from build123d import *

# Parameters (mm, degrees)
F1_DEPTH = 3.2
F2_R     = 14.060754
F3_DEPTH = 2


with BuildPart() as f1:
    # F0 (on Top) → F1 (new body)
    with BuildSketch(Plane.XY):
        with BuildLine():
            ThreePointArc((-5.086545, -8.556186), (-9.186545, 0.743814), (-5.086545, 10.043814))
            Line((-5.086545, 10.043814), (2.413455, 10.043814))
            ThreePointArc((2.413455, 10.043814), (5.286519, 6.166676), (6.491109, 1.493814))
            Line((6.491109, 1.493814), (8.494175, 1.493814))
            ThreePointArc((8.494175, 1.493814), (6.941519, 7.333341), (3.15704, 12.043814))
            Line((3.15704, 12.043814), (-5.83013, 12.043814))
            ThreePointArc((-5.83013, 12.043814), (-11.186545, 0.743814), (-5.83013, -10.556186))
            Line((-5.83013, -10.556186), (3.15704, -10.556186))
            ThreePointArc((3.15704, -10.556186), (6.941519, -5.845714), (8.494175, -0.006186))
            Line((8.494175, -0.006186), (6.491109, -0.006186))
            ThreePointArc((6.491109, -0.006186), (5.286519, -4.679049), (2.413455, -8.556186))
            Line((2.413455, -8.556186), (-5.086545, -8.556186))
        make_face()
    extrude(amount=F1_DEPTH)

    # F2 (on Top) → F3 (join)
    with BuildSketch(Plane.XY):
        with Locations((-1.336545, 0.743814)):
            Circle(F2_R)
    extrude(amount=-F3_DEPTH)


solid = f1.part
CAD build for the part. Positions are in the model's coordinates, mm. A direction names the side the tool comes from. Round coordinates to 2 decimals unless told otherwise and drop trailing zeros. Order: outer loops, then holes, each group sorted by start corner. A loop starts at its lowest first (then second) coordinate and runs counter-clockwise, first axis right, second up. Notation, with made-up numbers: (72.5, -17.5) -> (126.5, -17.5) arc R19 ccw to (126.5, -12.5) -> close; hole circle Ø3 at (-21, 1). An arc over 180 degrees is marked (long way). Write item = value, one per line. Start each with the question number.
(1) Cut at C-C, the plane z = 0.8. List the corners of the cut face in (x, y), then the cut area to 3 significant figures.
(2) Cut at A-A, the plane y = 11.25. List the corners of the cut face in (x, z).
(3) Which spindle directions (+Z, -Z, +X, -X, +Y, -Y) get a long thin tool onto all of the face, cutting with end or side? Do faces 4 (the cylindrical face through (-11.185, 0.925, 1.578)), 5 (the flat face through (-1, -10.556, 2)), 6 (the flat face through (7, 1.494, 2)), 7 (the cylindrical face through (-9.186, 0.597, 1.578)), 8 (the flat face through (-1, 12.044, 2)). Say none if no direction does.
(4) Cut at D-D, the plane x = -10.25. List the corners of the cut face in (y, z), then the cut area to 3 significant figures.
(5) Probe line 1 (Y direction, x = 5, z = 2.9); line 2 (Y direction, x = -0.25, z = 0.45); line 3 (X direction, y = 7.25, z = 0.6). List the from-to ranges inside material, lowest first. Write a range as [from, to].
(6) Cut at B-B, the plane x = -2.75. List the corners of the cut face in (y, z), then the cut area to 3 significant figures.
(7) Pull direction Y, two halves, no side cores. Call faces 1 (the flat face through (-9.4, 0.8, 3.2)), 2 (the cylindrical face through (6.98, 7.26, 1.58)), 3 (the flat face through (8, -0.006, 2)): released by +Y, released by -Y, zero draft, split by the parting line, or undercut.
(8) Pin check, flat tips, straight feed: P1, Ø2.5, axis at x = -1.5, z = 1.5, coming from the +Y side; P2, Ø0.6, axis at x = 7, z = 2, coming from the +Y side; P3, Ø1, axis at y = -2, z = -1, coming from the +X side. Stop position of each tip, or through.
Model answer:
q1.outline = (-5.83, -10.56) -> (3.16, -10.56) arc R14.6 ccw to (8.49, -0.01) -> (6.49, -0.01) arc R12.6 cw to (2.41, -8.56) -> (-5.09, -8.56) arc R12.6 cw to (-5.09, 10.04) -> (2.41, 10.04) arc R12.6 cw to (6.49, 1.49) -> (8.49, 1.49) arc R14.6 ccw to (3.16, 12.04) -> (-5.83, 12.04) arc R14.6 ccw to start
q1.area = 124 mm2
q2.outline = (-10.68, -2) -> (8.01, -2) -> (8.01, 0) -> (4.05, 0) -> (4.05, 3.2) -> (-6.72, 3.2) -> (-6.72, 0) -> (-10.68, 0) -> close
q3.face_4 = +Z, -X
q3.face_5 = +Z, +X, -X, -Y
q3.face_6 = +Z, +X
q3.face_7 = +Z
q3.face_8 = +Z, +X, -X, +Y
q4.outline = (-10.13, -2) -> (11.62, -2) -> (11.62, 0) -> (5.89, 0) -> (5.89, 3.2) -> (-4.4, 3.2) -> (-4.4, 0) -> (-10.13, 0) -> close
q4.area = 76.4 mm2
q5.line_1 = [-8.76, -5.24], [6.73, 10.24]
q5.line_2 = [-10.56, -8.56], [10.04, 12.04]
q5.line_3 = [-9.66, -7.38], [4.7, 6.98]
q6.outline = (-13.25, -2) -> (14.73, -2) -> (14.73, 0) -> (12.04, 0) -> (12.04, 3.2) -> (10.04, 3.2) -> (10.04, 0) -> (-8.56, 0) -> (-8.56, 3.2) -> (-10.56, 3.2) -> (-10.56, 0) -> (-13.25, 0) -> close
q6.area = 68.8 mm2
q7.face_1 = zero draft
q7.face_2 = released by +Y
q7.face_3 = undercut
q8.P1 = 12.04
q8.P2 = 7.79
q8.P3 = 12.54
